from build123d import *

# Parameters (mm, degrees)
F0_W     = 28
F0_H     = 28
F0_W_2   = 20
F0_H_2   = 20
F1_DEPTH = 40
F2_R     = 1.5
F3_R     = 5
F4_SIZE  = 1.5
F5_SIZE  = 0.5


with BuildPart() as f1:
    # F0 (on Top) → F1 (new body)
    with BuildSketch(Plane.XY):
        Rectangle(F0_W, F0_H)
        Rectangle(F0_W_2, F0_H_2, mode=Mode.SUBTRACT)
    extrude(amount=F1_DEPTH)

    # F2
    f2_edges = [f1.edges().sort_by_distance(p)[0] for p in [
        (-10, 10, 20),
        (10, 10, 20),
        (10, -10, 20),
        (-10, -10, 20),
    ]]
    fillet(f2_edges, radius=F2_R)

    # F3
    f3_edges = [f1.edges().sort_by_distance(p)[0] for p in [
        (-14, 14, 20),
        (-14, -14, 20),
        (14, -14, 20),
        (14, 14, 20),
    ]]
    fillet(f3_edges, radius=F3_R)

    # F4
    f4_edges = [f1.edges().sort_by_distance(p)[0] for p in [
        (-14, 0, 40),
        (-14, 0, 0),
    ]]
    chamfer(f4_edges, length=F4_SIZE)

    # F5
    f5_edges = [f1.edges().sort_by_distance(p)[0] for p in [
        (-10, 0, 40),
        (0, -10, 0),
    ]]
    chamfer(f5_edges, length=F5_SIZE)


solid = f1.part
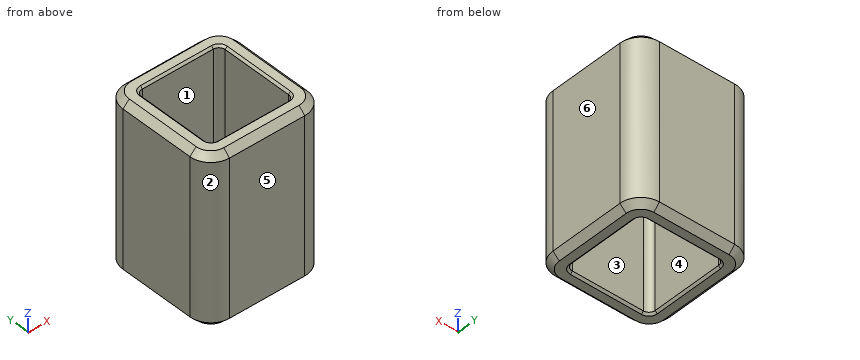
Geometry check sheet. Reference: the model listing, model coordinates, mm. Face numbers are marked on the shaded views. A direction names the side the tool comes from. Round coordinates to 2 decimals unless told otherwise and drop trailing zeros. Loops run counter-clockwise (first coordinate to the right, second up) from the corner with the lowest first, then second, coordinate; pieces in that order, holes last.
Item 1: Cross-section at C-C on z = 13. Record the boundary of the cut face in (x, y), then the cut area to 3 significant figures.
Item 2: Cross-section at A-A on x = 2. Record the boundary of the cut face in (y, z).
Item 3: Mould release check, pull along Y, two halves, no side actions. Record for the marked faces 3, 4, 5 and 6: pulls with the +Y half, pulls with the -Y half, needs draft (parallel to the pull), parting line crosses it, or undercut.
Item 4: Gauge pin test, flat end, axial feed: pin 1 (2 mm diameter, centred on y = 10, z = 7.5, fed in from -X). Record the tip position at first contact, or that the pin passes through.
Item 5: Thickness scan on line 1 (Y direction, x = -6.75, z = 24); line 2 (Y direction, x = 9.5, z = 15). Record the ranges inside material, lowest first.
Item 6: Access from +Z, -Z, +X, -X, +Y, -Y to the whole of each face (thin tool, end or side, straight path). Record for the marked faces 1 and 2.
Answer sheet:
1. outline: (-14, -9) arc R5 ccw to (-9, -14) - (9, -14) arc R5 ccw to (14, -9) - (14, 9) arc R5 ccw to (9, 14) - (-9, 14) arc R5 ccw to (-14, 9) - close; hole (-10, -8.5) arc R1.5 ccw to (-8.5, -10) - (8.5, -10) arc R1.5 ccw to (10, -8.5) - (10, 8.5) arc R1.5 ccw to (8.5, 10) - (-8.5, 10) arc R1.5 ccw to (-10, 8.5) - close
1. area: 364 mm2
2. outline: (-14, 1.5) - (-12.5, 0) - (-10.5, 0) - (-10, 0.5) - (-10, 39.5) - (-10.5, 40) - (-12.5, 40) - (-14, 38.5) - close; (10, 0.5) - (10.5, 0) - (12.5, 0) - (14, 1.5) - (14, 38.5) - (12.5, 40) - (10.5, 40) - (10, 39.5) - close
3. face 3: undercut
3. face 4: undercut
3. face 5: pulls with the -Y half
3. face 6: needs draft
4. pin 1: stops at x = -14
5. line 1: y = -14 to -10, 10 to 14
5. line 2: y = -13.97 to -9.62, 9.62 to 13.97
6. face 1: +Z, -Z
6. face 2: +Z, -Z, -X, -Y
